from build123d import *

# Parameters (mm, degrees)
SKETCH_1_W          = 90
SKETCH_1_H          = 150
EXTRUDE_1_DEPTH     = 3
CUT_EXTRUDE_1_DEPTH = 3
SKETCH_4_W          = 137
SKETCH_4_H          = 1.2
EXTRUDE_2_DEPTH     = 10
SKETCH_5_W          = 137
SKETCH_5_H          = 1.2
EXTRUDE_3_DEPTH     = 10
FILLET_1_R          = 3
SKETCH_6_R          = 1.5
CUT_EXTRUDE_2_DEPTH = 10
SKETCH_7_R          = 1.5
CUT_EXTRUDE_3_DEPTH = 10


with BuildPart() as part:
    # 草图1 → 凸台-拉伸1 (new body)
    with BuildSketch(Plane(origin=(0, 0, 0), x_dir=(1, 0, 0), z_dir=(0, 1, 0))):
        Rectangle(SKETCH_1_W, SKETCH_1_H)
    extrude(amount=EXTRUDE_1_DEPTH)

    # 草图2 → 切除-拉伸1 (cut)
    with BuildSketch(Plane(origin=(0, 3, 0), x_dir=(1, 0, 0), z_dir=(0, 1, 0))):
        with BuildLine():
            Line((-32.5, 40), (0, 40))
            Line((0, 40), (0, 45))
            Line((0, 45), (-27.5, 45))
            ThreePointArc((-27.5, 45), (-31.035533906, 43.535533906), (-32.5, 40))
        make_face()
        with BuildLine():
            Line((0, 45), (0, 40))
            Line((0, 40), (32.5, 40))
            ThreePointArc((32.5, 40), (31.035533906, 43.535533906), (27.5, 45))
            Line((27.5, 45), (0, 45))
        make_face()
        with BuildLine():
            Line((-27.5, 35), (0, 35))
            Line((0, 35), (0, 40))
            Line((0, 40), (-32.5, 40))
            ThreePointArc((-32.5, 40), (-31.035533906, 36.464466094), (-27.5, 35))
        make_face()
        with BuildLine():
            Line((0, 40), (0, 35))
            Line((0, 35), (27.5, 35))
            ThreePointArc((27.5, 35), (31.035533906, 36.464466094), (32.5, 40))
            Line((32.5, 40), (0, 40))
        make_face()
        with BuildLine():
            ThreePointArc((-27.5, 5), (-31.035533906, 3.535533906), (-32.5, 0))
            Line((-32.5, 0), (0, 0))
            Line((0, 0), (0, 5))
            Line((0, 5), (-27.5, 5))
        make_face()
        with BuildLine():
            Line((0, 5), (0, 0))
            Line((0, 0), (32.5, 0))
            ThreePointArc((32.5, 0), (31.035533906, 3.535533906), (27.5, 5))
            Line((27.5, 5), (0, 5))
        make_face()
        with BuildLine():
            Line((32.5, 0), (0, 0))
            Line((0, 0), (0, -5))
            Line((0, -5), (27.5, -5))
            ThreePointArc((27.5, -5), (31.035533906, -3.535533906), (32.5, 0))
        make_face()
        with BuildLine():
            Line((0, 0), (-32.5, 0))
            ThreePointArc((-32.5, 0), (-31.035533906, -3.535533906), (-27.5, -5))
            Line((-27.5, -5), (0, -5))
            Line((0, -5), (0, 0))
        make_face()
        with BuildLine():
            Line((0, -40), (0, -35))
            Line((0, -35), (-27.5, -35))
            ThreePointArc((-27.5, -35), (-31.035533906, -36.464466094), (-32.5, -40))
            Line((-32.5, -40), (0, -40))
        make_face()
        with BuildLine():
            Line((27.5, -35), (0, -35))
            Line((0, -35), (0, -40))
            Line((0, -40), (32.5, -40))
            ThreePointArc((32.5, -40), (31.035533906, -36.464466094), (27.5, -35))
        make_face()
        with BuildLine():
            Line((0, -45), (0, -40))
            Line((0, -40), (-32.5, -40))
            ThreePointArc((-32.5, -40), (-31.035533906, -43.535533906), (-27.5, -45))
            Line((-27.5, -45), (0, -45))
        make_face()
        with BuildLine():
            Line((32.5, -40), (0, -40))
            Line((0, -40), (0, -45))
            Line((0, -45), (27.5, -45))
            ThreePointArc((27.5, -45), (31.035533906, -43.535533906), (32.5, -40))
        make_face()
    extrude(amount=-CUT_EXTRUDE_1_DEPTH, mode=Mode.SUBTRACT)

    # 草图4 → 凸台-拉伸2 (add)
    with BuildSketch(Plane(origin=(45, 0, 0), x_dir=(0, 0, -1), z_dir=(1, 0, 0))):
        with Locations((0, 0.9)):
            Rectangle(SKETCH_4_W, SKETCH_4_H)
        with Locations((0, 2.1)):
            Rectangle(SKETCH_4_W, SKETCH_4_H)
    extrude(amount=EXTRUDE_2_DEPTH)

    # 草图5 → 凸台-拉伸3 (add)
    with BuildSketch(Plane.ZY.offset(45)):
        with Locations((0, 2.1)):
            Rectangle(SKETCH_5_W, SKETCH_5_H)
        with Locations((0, 0.9)):
            Rectangle(SKETCH_5_W, SKETCH_5_H)
    extrude(amount=EXTRUDE_3_DEPTH)

    # 圆角1
    fillet_1_edges = [part.edges().sort_by_distance(p)[0] for p in [
        (55, 1.5, -68.5),
        (55, 1.5, 68.5),
        (-55, 1.5, 68.5),
        (-55, 1.5, -68.5),
    ]]
    fillet(fillet_1_edges, radius=FILLET_1_R)

    # 草图6 → 切除-拉伸2 (cut)
    with BuildSketch(Plane(origin=(0, 2.7, 0), x_dir=(1, 0, 0), z_dir=(0, 1, 0))):
        with Locations((50, 0)):
            Circle(SKETCH_6_R)
    extrude(amount=-CUT_EXTRUDE_2_DEPTH, mode=Mode.SUBTRACT)

    # 草图7 → 切除-拉伸3 (cut)
    with BuildSketch(Plane(origin=(0, 2.7, 0), x_dir=(1, 0, 0), z_dir=(0, 1, 0))):
        with Locations((-50, 0)):
            Circle(SKETCH_7_R)
    extrude(amount=-CUT_EXTRUDE_3_DEPTH, mode=Mode.SUBTRACT)


solid = part.part
Build history of the part. All positions in model axes, mm. A direction names the side the tool comes from. Round coordinates to 2 decimals unless told otherwise and drop trailing zeros. Loops run counter-clockwise (first coordinate to the right, second up) from the corner with the lowest first, then second, coordinate; pieces in that order, holes last. Notation, with made-up numbers: (-14.5, 87) -> (35.5, 87) arc R11 ccw to (35.5, 106) -> close; hole circle Ø6 at (43, 24.25). An arc over 180 degrees is marked (long way). Answer in a Markdown table with one row per item.
Item 1: Which spindle directions (+Z, -Z, +X, -X, +Y, -Y) get a long thin tool onto all of the face, cutting with end or side? Do faces 1 (the flat face through (0, 2, 45)), 2 (the flat face through (-48, 2.7, -1)), 3 (the flat face through (48, 0.3, 1)), 4 (the flat face through (48, 2.7, 1)), 5 (the flat face through (-1, 1, -75)). Say none if no direction does.
Answers below:
| item | result |
|---|---|
| face 1 | +Y, -Y |
| face 2 | +Z, -Z, -X, +Y |
| face 3 | +Z, -Z, +X, -Y |
| face 4 | +Z, -Z, +X, +Y |
| face 5 | -Z, +X, -X, +Y, -Y |
Item 2: Drill centre lines: L1, parallel to Z at x = 20.5, y = 2; L2, parallel to Z at x = 50, y = 1.85; L3, parallel to Z at x = -29, y = 2. Where is each one in solid material? Low to high. Write a range as [from, to].
Answers below:
| item | result |
|---|---|
| L1 | z = [-75, -45], [-35, -5], [5, 35], [45, 75] |
| L2 | z = [-68.5, -1.5], [1.5, 68.5] |
| L3 | z = [-75, -44.77], [-35.23, -4.77], [4.77, 35.23], [44.77, 75] |
Item 3: Saw through at A-A (x = 50). Write the cut outline in (y, z), and give its area (3 significant figures).
Answers below:
| item | result |
|---|---|
| outline | (0.3, -68.5) -> (2.7, -68.5) -> (2.7, -1.5) -> (0.3, -1.5) -> close; (0.3, 1.5) -> (2.7, 1.5) -> (2.7, 68.5) -> (0.3, 68.5) -> close |
| area | 322 mm² |
Item 4: Mould opens along X. For faces 6 (the cylindrical face through (54.1, 1.48, 67.64)), 7 (the cylindrical face through (-51.5, 1.52, -0.07)), 8 (the flat face through (-48, 0.3, -1)) say: +X half, -X half, draft (parallel to the pull), parting line (faces both ways), or undercut.
Answers below:
| item | result |
|---|---|
| face 6 | +X half |
| face 7 | undercut |
| face 8 | draft |
Item 5: Saw through at C-C (z = 29). Write the cut outline in (x, y), and give its area (3 significant figures).
Answers below:
| item | result |
|---|---|
| outline | (-55, 0.3) -> (-45, 0.3) -> (-45, 0) -> (45, 0) -> (45, 0.3) -> (55, 0.3) -> (55, 2.7) -> (45, 2.7) -> (45, 3) -> (-45, 3) -> (-45, 2.7) -> (-55, 2.7) -> close |
| area | 318 mm² |
Item 6: Saw through at D-D (y = 2). State how many separate pieces and enclosed holes the cut face has, and give its area (3 significant figures).
Answers below:
| item | result |
|---|---|
| separate pieces | 1 |
| enclosed holes | 5 |
| area | 14,300 mm² |
Item 7: Saw through at B-B (x = 0). Write the cut outline in (y, z), and give its area (3 significant figures).
Answers below:
| item | result |
|---|---|
| outline | (0, -75) -> (3, -75) -> (3, -45) -> (0, -45) -> close; (0, -35) -> (3, -35) -> (3, -5) -> (0, -5) -> close; (0, 5) -> (3, 5) -> (3, 35) -> (0, 35) -> close; (0, 45) -> (3, 45) -> (3, 75) -> (0, 75) -> close |
| area | 360 mm² |
Item 8: Pin check, flat tips, straight feed: pin 1 (6 mm diameter, centred on x = 8, z = 59.5, fed in from -Y); pin 2 (0.7 mm diameter, centred on x = -47.5, y = 1.5, fed in from -Z); pin 3 (2.5 mm diameter, centred on x = 50, z = 0, fed in from +Y); pin 4 (8 mm diameter, centred on x = 50, z = 31, fed in from +Y). Stop position of each tip, or through.
Answers below:
| item | result |
|---|---|
| pin 1 | stops at y = 0 |
| pin 2 | stops at z = -68.5 |
| pin 3 | passes through |
| pin 4 | stops at y = 2.7 |
